Read the model definition and answer for the solid it produces. Units are mm, in the model's axes. Face numbers are marked on the shaded views. A direction names the side the tool comes from. Coordinates: 2 decimals unless noted, no trailing zeros. Write each loop counter-clockwise with the first axis right and the second up, starting at its lowest first coordinate (ties: lowest second). Pieces come first, ordered by that corner, then holes.
Autodesk Inventor part; units mm, degrees
ref_plane "Work Plane1" through (30, 0, 0) normal (0, -0.5, 0.866) x (1, 0, 0)
ref_plane "YZ Plane" through (0, 0, 0) normal (1, 0, 0) x (0, 1, 0)
ref_plane "XZ Plane" through (0, 0, 0) normal (0, 1, 0) x (-1, 0, 0)
sketch "Sketch1" plane through (0, 0, 0) normal (0, 0, 1) x (1, 0, 0)
  line L0 (0.0567, 0) -> (12, 0)
  line L1 (12, 0) -> (12, 1.5)
  line L2 (12, 1.5) -> (1, 1.5)
  line L3 (1, 1.5) -> (0.6933, 1.5)
  line L4 (0.6933, 1.5) -> (0, 1.5)
  line L5 (0, 1.5) -> (0, 2.85)
  line L6 (0, 2.85) -> (-1.65, 2.85)
  line L7 (-1.65, 2.85) -> (-1.65, 1.1547)
  line L8 (-1.65, 1.1547) -> (-0.61, 1.1547)
  line L9 (-0.61, 1.1547) -> (0.0567, 0)
  line L10 (-4.38, 0) -> (14.73, 0)
  line L11 (0, -0.57) -> (0, 3.42)
  line L12 (1, 1.5) -> (0, 1.5) construction
  dimension "d0" = 11
  dimension "d1" = 0.3067
  dimension "d2" = 1.65
  dimension "d3" = 1.04
  dimension "d4" = 60
  dimension "d5" = 3
  dimension "d6" = 3
  dimension "d7" = 2.3094
  dimension "d8" = 5.7
  dimension "d19" = 12
revolve "Body" add sketch "Sketch1" angle 360 about axis through (0.0567, 0, 0) along (1, 0, 0) contours L9 L11 L4 L3 L2 L1 L0 | L9 L8 L7 L6 L5 L11
sketch "Sketch2" plane through (-1.65, 0, 0) normal (-1, 0, 0) x (0, 0, 1)
  circle A0 centre (0, 0) radius 1.1547
  line L0 (0, -3.99) -> (0, 3.99)
  line L1 (-3.99, 0) -> (3.99, 0)
  line L2 (1.1547, 0) -> (0.5774, -1)
  line L3 (0.5774, -1) -> (-0.5774, -1)
  line L4 (-0.5774, -1) -> (-1.1547, 0)
  line L5 (-1.1547, 0) -> (-0.5774, 1)
  line L6 (-0.5774, 1) -> (0.5774, 1)
  line L7 (0.5774, 1) -> (1.1547, 0)
extrude "Slot" add sketch "Sketch2" against normal up to next contours L7 A0 | A0 L2 | L6 L0 A0 | A0 L0 L3 | L0 L6 A0 | A0 L3 L0 | L4 A0 | A0 L5
fillet "Fillet1" radius 1.425 1 edges at (-1.65, -2.85, 0)
thread "Thread"
chamfer "Chamfer1" distance 0.3067 distance2 0.3067 1 edges at (12, -1.5, 0) measured on face at (12, -0.6587, -0.1791)
fillet "Fillet2" radius 0.1 1 edges at (0, -1.5, 0)
ref_plane "Work Plane1" through (30, 0, 0) normal (0, -0.5, 0.866) x (1, 0, 0)
equation "\"d0\" = GEL"
equation "\"d1\" = GAL"
equation "\"d2\" = KOH"
equation "\"d3\" = INTI"
equation "\"d5\" = GD"
equation "\"d6\" = BDM"
equation "\"d7\" = 1.1547 * SW"
equation "\"d8\" = KOD"
equation "\"d19\" = NLG"
equation "\"d16\" = RR"
equation "\"d12\" = GEL"
equation "\"d14\" = -0.5 * SPD + 0.5 * GD"
equation "\"d15\" = GUL"
equation "\"d29\" = R"
equation "\"GD\" = NND"
equation "\"NLG\" = 12"
equation "\"GEL\" = 11"
equation "\"KOD\" = 5.7"
equation "\"KOH\" = 1.65"
equation "\"INTI\" = 1.04"
equation "\"GAL\" = 0.61345 * PTC"
equation "\"GUL\" = 0.61345 * PTC"
equation "\"BDM\" = NND"
equation "\"SW\" = 2"
equation "\"RR\" = 1.425"
equation "\"SPD\" = 2.38655"
equation "\"d28\" = R"
equation "\"R\" = 0.1"
equation "\"TOA\" = 30deg"
equation "\"THREADDIA\" = 3"
equation "\"KOD1\" = KOD - 2 * RR"
equation "\"PTC\" = 0.5"
equation "\"NND\" = 3"
equation "\"E0\" = 1.155 * SW"
equation "\"GD1\" = THREADDIA - 1.2269 * PTC"
properties part number "ANSI B18.3.4M - M3 x 0.5 x 12" material "Steel, Mild"
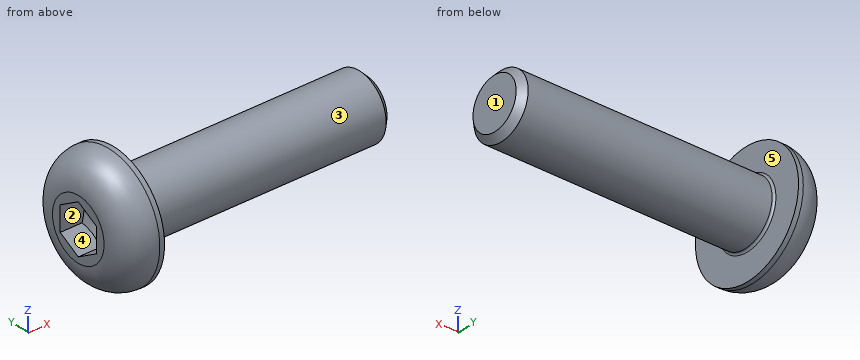
Item 1: The part is cut by section A-A (x = 2.5). Give the vertices of the cut face in (y, z), and give its area (3 significant figures).
Item 2: Given pin 1 (3 mm diameter, centred on x = 10, z = -1.5, fed in from -Y); pin 2 (3 mm diameter, centred on x = 3.5, y = 1, fed in from +Z); pin 3 (3 mm diameter, centred on x = 3.5, z = -0.5, fed in from +Y), each flat-ended and moving along its own axis, determine where each tip first touches the part or whether it passes through.
Item 3: For the marked faces 1 and 2, determine the directions among +Z, -Z, +X, -X, +Y, -Y from which every point of the face is accessible in a straight line to the end or side of a thin tool.
Item 4: Find the intervals of material crossed by probe 1 along Z at (x, y) = (-0.5, 0.2); probe 2 along X at (y, z) = (-2.4, -1.1); probe 3 along Z at (x, y) = (6, 1.05), in increasing order.
Item 5: Determine the mould class of the marked faces 3, 4 and 5 for opening direction Z: +Z half, -Z half, draft (parallel to the pull), parting line (faces both ways), or undercut.
Answer:
1. outline: circle Ø3 at (0, 0)
1. area: 7.07 mm2
2. pin 1: stops at y = -1.5
2. pin 2: stops at z = 1.5
2. pin 3: stops at y = 1.5
3. face 1: +Z, -Z, +X, +Y, -Y
3. face 2: -X
4. probe 1: z = -2.82 to -0.94, 0.94 to 2.82
4. probe 2: x = -0.97 to 0
4. probe 3: z = -1.07 to 1.07
5. face 3: parting line
5. face 4: undercut
5. face 5: draft
